Design review of the part built by this model. Coordinates are the model's own, in mm. Round coordinates to 2 decimals unless told otherwise and drop trailing zeros. Write each loop counter-clockwise with the first axis right and the second up, starting at its lowest first coordinate (ties: lowest second). Pieces come first, ordered by that corner, then holes. Notation, with made-up numbers: M 7,-3.5 L 36,-3.5 A30 cw 36,30.5 Z; hole C 62,26.25 d2. An arc over 180 degrees is marked long. Use CSV: the item, a comma, the result in double quotes.
from build123d import *

# Parameters (mm, degrees)
BOSS_EXTRUDE1_DEPTH = 7.5
SKETCH1_3_R         = 20
BOSS_EXTRUDE2_DEPTH = 5


with BuildPart() as part:
    # Sketch1 → Boss-Extrude1 (new, symmetric)
    with BuildSketch(Plane.XY):
        with BuildLine():
            ThreePointArc((-27.399817518, 11.5), (-25.852186654, 11.930011924), (-24.748222274, 13.096774194))
            ThreePointArc((-24.748222274, 13.096774194), (0, 28), (24.748222274, 13.096774194))
            ThreePointArc((24.748222274, 13.096774194), (25.852186654, 11.930011924), (27.399817518, 11.5))
            Line((27.399817518, 11.5), (35, 11.5))
            Line((35, 11.5), (35, -11.5))
            Line((35, -11.5), (27.399817518, -11.5))
            ThreePointArc((27.399817518, -11.5), (25.852186654, -11.930011924), (24.748222274, -13.096774194))
            ThreePointArc((24.748222274, -13.096774194), (0, -28), (-24.748222274, -13.096774194))
            ThreePointArc((-24.748222274, -13.096774194), (-25.852186654, -11.930011924), (-27.399817518, -11.5))
            Line((-27.399817518, -11.5), (-35, -11.5))
            Line((-35, -11.5), (-35, 11.5))
            Line((-35, 11.5), (-27.399817518, 11.5))
        make_face()
        with BuildLine():
            ThreePointArc((27.399817518, 6.5), (23.272801881, 7.646698465), (20.328896868, 10.758064516))
            ThreePointArc((20.328896868, 10.758064516), (0, 23), (-20.328896868, 10.758064516))
            ThreePointArc((-20.328896868, 10.758064516), (-23.272801881, 7.646698465), (-27.399817518, 6.5))
            Line((-27.399817518, 6.5), (-30, 6.5))
            Line((-30, 6.5), (-30, -6.5))
            Line((-30, -6.5), (-27.399817518, -6.5))
            ThreePointArc((-27.399817518, -6.5), (-23.272801881, -7.646698465), (-20.328896868, -10.758064516))
            ThreePointArc((-20.328896868, -10.758064516), (0, -23), (20.328896868, -10.758064516))
            ThreePointArc((20.328896868, -10.758064516), (23.272801881, -7.646698465), (27.399817518, -6.5))
            Line((27.399817518, -6.5), (30, -6.5))
            Line((30, -6.5), (30, 6.5))
            Line((30, 6.5), (27.399817518, 6.5))
        make_face(mode=Mode.SUBTRACT)
    extrude(amount=BOSS_EXTRUDE1_DEPTH, both=True)

    # Sketch1_3 → Boss-Extrude2 (add, symmetric)
    with BuildSketch(Plane.XY):
        with BuildLine():
            Line((48.38539126, 39.482324053), (63.561930641, 48.24450315))
            ThreePointArc((63.561930641, 48.24450315), (64.74439519, 49.499305768), (65.040826193, 51.197799419))
            ThreePointArc((65.040826193, 51.197799419), (120.810543828, 69.75), (76.859008012, 30.728108057))
            ThreePointArc((76.859008012, 30.728108057), (75.23985386, 31.320638103), (73.561930641, 30.923995074))
            Line((73.561930641, 30.923995074), (58.38539126, 22.161815977))
            ThreePointArc((58.38539126, 22.161815977), (57.083792338, 20.636606711), (57.033705962, 18.63213311))
            ThreePointArc((57.033705962, 18.63213311), (60, 0), (57.033705962, -18.63213311))
            ThreePointArc((57.033705962, -18.63213311), (57.083792338, -20.636606711), (58.38539126, -22.161815977))
            Line((58.38539126, -22.161815977), (73.561930641, -30.923995074))
            ThreePointArc((73.561930641, -30.923995074), (75.23985386, -31.320638103), (76.859008012, -30.728108057))
            ThreePointArc((76.859008012, -30.728108057), (120.810543828, -69.75), (65.040826193, -51.197799419))
            ThreePointArc((65.040826193, -51.197799419), (64.74439519, -49.499305768), (63.561930641, -48.24450315))
            Line((63.561930641, -48.24450315), (48.38539126, -39.482324053))
            ThreePointArc((48.38539126, -39.482324053), (46.413721828, -39.117710954), (44.652753581, -40.07657168))
            ThreePointArc((44.652753581, -40.07657168), (30, -51.961524227), (12.380952381, -58.70870479))
            ThreePointArc((12.380952381, -58.70870479), (10.67007051, -59.754317665), (10, -61.64414003))
            Line((10, -61.64414003), (10, -79.168498224))
            ThreePointArc((10, -79.168498224), (10.49545867, -80.819943871), (11.818181818, -81.925907476))
            ThreePointArc((11.818181818, -81.925907476), (0, -139.5), (-11.818181818, -81.925907476))
            ThreePointArc((-11.818181818, -81.925907476), (-10.49545867, -80.819943871), (-10, -79.168498224))
            Line((-10, -79.168498224), (-10, -61.64414003))
            ThreePointArc((-10, -61.64414003), (-10.67007051, -59.754317665), (-12.380952381, -58.70870479))
            ThreePointArc((-12.380952381, -58.70870479), (-30, -51.961524227), (-44.652753581, -40.07657168))
            ThreePointArc((-44.652753581, -40.07657168), (-46.413721828, -39.117710954), (-48.38539126, -39.482324053))
            Line((-48.38539126, -39.482324053), (-63.561930641, -48.24450315))
            ThreePointArc((-63.561930641, -48.24450315), (-64.74439519, -49.499305768), (-65.040826193, -51.197799419))
            ThreePointArc((-65.040826193, -51.197799419), (-120.810543828, -69.75), (-76.859008012, -30.728108057))
            ThreePointArc((-76.859008012, -30.728108057), (-75.23985386, -31.320638103), (-73.561930641, -30.923995074))
            Line((-73.561930641, -30.923995074), (-58.38539126, -22.161815977))
            ThreePointArc((-58.38539126, -22.161815977), (-57.083792338, -20.636606711), (-57.033705962, -18.63213311))
            ThreePointArc((-57.033705962, -18.63213311), (-60, 0), (-57.033705962, 18.63213311))
            ThreePointArc((-57.033705962, 18.63213311), (-57.083792338, 20.636606711), (-58.38539126, 22.161815977))
            Line((-58.38539126, 22.161815977), (-73.561930641, 30.923995074))
            ThreePointArc((-73.561930641, 30.923995074), (-75.23985386, 31.320638103), (-76.859008012, 30.728108057))
            ThreePointArc((-76.859008012, 30.728108057), (-120.308802103, 70.587282596), (-65.334884287, 49.268118414))
            Line((-65.334884287, 49.268118414), (-48.38539126, 39.482324053))
            ThreePointArc((-48.38539126, 39.482324053), (-46.413721828, 39.117710954), (-44.652753581, 40.07657168))
            ThreePointArc((-44.652753581, 40.07657168), (-30, 51.961524227), (-12.380952381, 58.70870479))
            ThreePointArc((-12.380952381, 58.70870479), (-10.67007051, 59.754317665), (-10, 61.64414003))
            Line((-10, 61.64414003), (-10, 79.168498224))
            ThreePointArc((-10, 79.168498224), (-10.49545867, 80.819943871), (-11.818181818, 81.925907476))
            ThreePointArc((-11.818181818, 81.925907476), (0, 139.5), (11.818181818, 81.925907476))
            ThreePointArc((11.818181818, 81.925907476), (10.49545867, 80.819943871), (10, 79.168498224))
            Line((10, 79.168498224), (10, 61.64414003))
            ThreePointArc((10, 61.64414003), (10.67007051, 59.754317665), (12.380952381, 58.70870479))
            ThreePointArc((12.380952381, 58.70870479), (30, 51.961524227), (44.652753581, 40.07657168))
            ThreePointArc((44.652753581, 40.07657168), (46.413721828, 39.117710954), (48.38539126, 39.482324053))
        make_face()
        with Locations((94.829781714, 54.75)):
            Circle(SKETCH1_3_R, mode=Mode.SUBTRACT)
        with Locations((94.829781714, -54.75)):
            Circle(SKETCH1_3_R, mode=Mode.SUBTRACT)
        with Locations((0, -109.5)):
            Circle(SKETCH1_3_R, mode=Mode.SUBTRACT)
        with Locations((-94.829781714, -54.75)):
            Circle(SKETCH1_3_R, mode=Mode.SUBTRACT)
        with Locations((-94.829781714, 54.75)):
            Circle(SKETCH1_3_R, mode=Mode.SUBTRACT)
        with Locations((0, 109.5)):
            Circle(SKETCH1_3_R, mode=Mode.SUBTRACT)
        with BuildLine():
            Line((-27.399817518, 11.5), (-35, 11.5))
            Line((-35, 11.5), (-35, -11.5))
            Line((-35, -11.5), (-27.399817518, -11.5))
            ThreePointArc((-27.399817518, -11.5), (-25.852186654, -11.930011924), (-24.748222274, -13.096774194))
            ThreePointArc((-24.748222274, -13.096774194), (0, -28), (24.748222274, -13.096774194))
            ThreePointArc((24.748222274, -13.096774194), (25.852186654, -11.930011924), (27.399817518, -11.5))
            Line((27.399817518, -11.5), (35, -11.5))
            Line((35, -11.5), (35, 11.5))
            Line((35, 11.5), (27.399817518, 11.5))
            ThreePointArc((27.399817518, 11.5), (25.852186654, 11.930011924), (24.748222274, 13.096774194))
            ThreePointArc((24.748222274, 13.096774194), (0, 28), (-24.748222274, 13.096774194))
            ThreePointArc((-24.748222274, 13.096774194), (-25.852186654, 11.930011924), (-27.399817518, 11.5))
        make_face(mode=Mode.SUBTRACT)
    extrude(amount=BOSS_EXTRUDE2_DEPTH, both=True)


solid = part.part
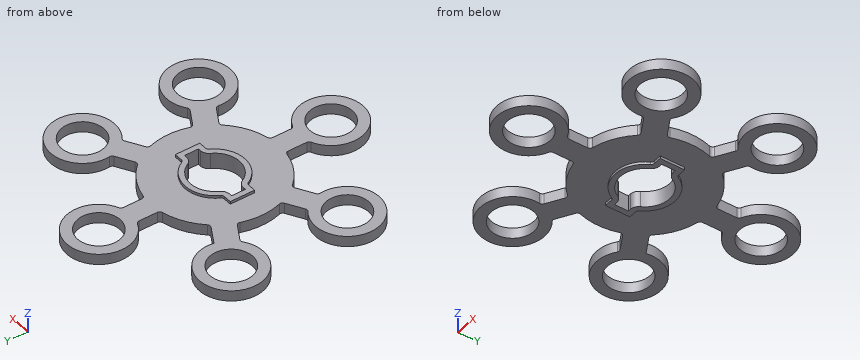
1) Add section D-D on z = 0.5. Give the number of separate pieces and of enclosed holes in the cut face, then the cut area to 3 significant figures.
Answers:
separate pieces,"1"
enclosed holes,"7"
area,"21,300 mm²"
2) Wall thickness on line 1 along X through (y, z) = (-52, -4); line 2 along Y through (x, z) = (-25, -3); line 3 along X through (y, z) = (79, 0.5): over which ranges is each line inside the solid? List them lowest first. Write a range as [from, to].
Answers:
line 1,"[-124.7, -114.64], [-75.02, -64.96], [-29.93, 29.93], [64.96, 75.02], [114.64, 124.7]"
line 2,"[-126.08, -92.92], [-54.54, -6.87], [6.87, 54.54], [92.92, 126.08]"
line 3,"[-112.49, -77.17], [-10, 10], [77.17, 112.49]"
3) For pin 1 Ø8 at (y, z) = (24, -5.5) entering from +X; pin 2 Ø10 at (x, y) = (-62.5, -51) entering from -Z; pin 3 Ø5 at (x, y) = (-80.5, -45.5) entering from -Z; pin 4 Ø3 at (y, z) = (3.5, 5.5) entering from +X, all flat-tipped, find the tip position at first contact; note any pin that passes through.
Answers:
pin 1,"x = 108.35"
pin 2,"z = -5"
pin 3,"through"
pin 4,"x = 59.96"
4) Add section A-A on y = 109.5. Write out the cut boundary in (x, z), then the cut area to 3 significant figures.
Answers:
outline,"M -30,-5 L -20,-5 L -20,5 L -30,5 Z; M 20,-5 L 30,-5 L 30,5 L 20,5 Z"
area,"200 mm²"
5) Add section B-B on y = -54.75. Write out the cut boundary in (x, z), then the cut area to 3 significant figures.
Answers:
outline,"M -124.83,-5 L -114.83,-5 L -114.83,5 L -124.83,5 Z; M -74.83,-5 L -64.83,-5 L -64.83,5 L -74.83,5 Z; M -24.54,-5 L 24.54,-5 L 24.54,5 L -24.54,5 Z; M 64.83,-5 L 74.83,-5 L 74.83,5 L 64.83,5 Z; M 114.83,-5 L 124.83,-5 L 124.83,5 L 114.83,5 Z"
area,"891 mm²"
6) Add section C-C on y = -104. Write out the cut boundary in (x, z), then the cut area to 3 significant figures.
Answers:
outline,"M -29.49,-5 L -19.23,-5 L -19.23,5 L -29.49,5 Z; M 19.23,-5 L 29.49,-5 L 29.49,5 L 19.23,5 Z"
area,"205 mm²"
